Could you check a few things on this model? Use its own coordinates, in mm. Coordinates: 2 decimals unless noted, no trailing zeros. Answer as CSV lines item,"result". Start each with the question number.
Item 1: We'd pull the mould along Z, two halves only. Please class faces 1 (the cylindrical face through (-156.32, -3.13, 61.33)), 2 (the flat face through (-186.006, -3, -1)), 3 (the flat face through (-11, -3, 76.2)), 4 (the flat face through (-11, -3, -76.2)): +Z half, -Z half, draft (parallel to the pull), parting line (faces both ways), or undercut.
Item 2: If I drill on line 1 along Z through (x, y) = (0, -2); line 2 along X through (y, z) = (-5, 7.5); line 3 along Z through (x, y) = (142, -3.5), over which ranges is the centre line in solid material (lowest first)? Write a range as [from, to].
Item 3: I'm going to push a flat-ended pin straight in: P1, Ø2, axis at x = 0, z = -7.62, coming from the -Y side. Where does the tip first touch, or does it pass through?
```python
from build123d import *

# Parameters (mm, degrees)
F0_W     = 355.6
F0_H     = 152.4
F1_DEPTH = 6.35
F3_D     = 2.54
F5_D     = 7.62
F6_R     = 5.08
F8_D     = 2.54
F10_D    = 7.62
F12_D    = 7.62
F14_D    = 7.62
F16_D    = 7.62


with BuildPart() as f1:
    # F0 (on Front) → F1 (new body)
    with BuildSketch(Plane.XZ):
        with Locations((-8.206145, 0)):
            Rectangle(F0_W, F0_H)
    extrude(amount=F1_DEPTH)

    # F3 (through all)
    with Locations(Plane.XZ.offset(6.35)):
        with Locations((-7.62, 0), (0, 7.62), (7.62, 0), (0, -7.62)):
            Hole(F3_D / 2)

    # F5 (through all)
    with Locations(Plane.XZ.offset(6.35)):
        with Locations((0, 0), (111.570381, -56.575853), (138.698444, 61.264154)):
            Hole(F5_D / 2)

    # F6
    f6_edges = [f1.edges().sort_by_distance(p)[0] for p in [
        (169.593855, -3.175, 76.2),
        (169.593855, -3.175, -76.2),
        (-186.006145, -3.175, 76.2),
        (-186.006145, -3.175, -76.2),
    ]]
    fillet(f6_edges, radius=F6_R)

    # F8 (through all)
    with Locations(Plane.XZ.offset(6.35)):
        with Locations((111.570381, -48.955853), (117.046016, -51.276625), (119.190381, -56.575853), (117.237232, -61.670084), (111.570381, -64.195853), (106.344404, -62.121443), (103.950381, -56.575853), (106.327029, -51.046689)):
            Hole(F8_D / 2)

    # F10 (through all)
    with Locations(Plane.XZ.offset(6.35)):
        with Locations((-156.609148, -54.899529)):
            Hole(F10_D / 2)

    # F12 (through all)
    with Locations(Plane.XZ.offset(6.35)):
        with Locations((73.532805, 58.796812), (-160.125718, 61.164971)):
            Hole(F12_D / 2)

    # F14 (through all)
    with Locations(Plane.XZ.offset(6.35)):
        with Locations((-91.046117, 59.276842)):
            Hole(F14_D / 2)

    # F16 (through all)
    with Locations(Plane.XZ.offset(6.35)):
        with Locations((0, 56.724396)):
            Hole(F16_D / 2)


solid = f1.part
```
Ans:
1,face 1,"undercut"
1,face 2,"draft"
1,face 3,"+Z half"
1,face 4,"-Z half"
2,line 1,"z = [-76.2, -8.89], [-6.35, -3.81], [3.81, 6.35], [8.89, 52.91], [60.53, 76.2]"
2,line 2,"x = [-186.01, -1.26], [1.26, 169.59]"
2,line 3,"z = [-76.2, 59.36], [63.17, 76.2]"
3,P1,"passes through"
